For this review, take the finished solid that the model builds, in its own axes (mm). Round coordinates to 2 decimals unless told otherwise and drop trailing zeros. Write each loop counter-clockwise with the first axis right and the second up, starting at its lowest first coordinate (ties: lowest second). Pieces come first, ordered by that corner, then holes. Notation, with made-up numbers: M 61.25,70 L 103.25,70 A13 cw 103.25,88 Z; hole C 30,-11.75 d3. An arc over 180 degrees is marked long. One line per question, with ' | ' between items.
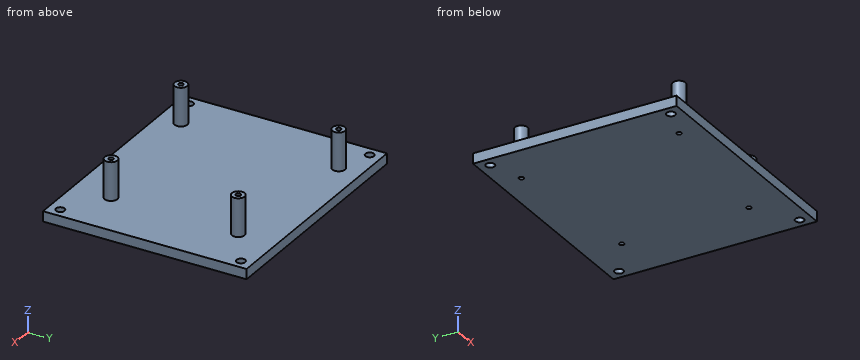
```python
from build123d import *

# Parameters (mm, degrees)
SKETCH_1_W          = 94
SKETCH_1_H          = 80
EXTRUDE_1_DEPTH     = 4
CUT_EXTRUDE_1_REACH = 63.847
SKETCH_2_R          = 1.7
SKETCH_3_R          = 2.5
EXTRUDE_2_DEPTH     = 15
CUT_EXTRUDE_2_REACH = 66.576
SKETCH_4_R          = 0.95


with BuildPart() as part:
    # 草图1 → 凸台-拉伸1 (new body)
    with BuildSketch(Plane.XY):
        Rectangle(SKETCH_1_W, SKETCH_1_H)
    extrude(amount=EXTRUDE_1_DEPTH)

    # 草图2 → 切除-拉伸1 (cut, up to next)
    with BuildSketch(Plane.XY.offset(4), mode=Mode.PRIVATE) as cut_extrude_1_sk1:
        with Locations((-43.1, -35.5)):
            Circle(SKETCH_2_R)
    cut_extrude_1_tool1 = extrude(cut_extrude_1_sk1.sketch, amount=-CUT_EXTRUDE_1_REACH, mode=Mode.PRIVATE) & part.part
    # 草图2 → 切除-拉伸1 (cut, up to next)
    with BuildSketch(Plane.XY.offset(4), mode=Mode.PRIVATE) as cut_extrude_1_sk2:
        with Locations((43.1, -35.5)):
            Circle(SKETCH_2_R)
    cut_extrude_1_tool2 = extrude(cut_extrude_1_sk2.sketch, amount=-CUT_EXTRUDE_1_REACH, mode=Mode.PRIVATE) & part.part
    # 草图2 → 切除-拉伸1 (cut, up to next)
    with BuildSketch(Plane.XY.offset(4), mode=Mode.PRIVATE) as cut_extrude_1_sk3:
        with Locations((43.1, 35.5)):
            Circle(SKETCH_2_R)
    cut_extrude_1_tool3 = extrude(cut_extrude_1_sk3.sketch, amount=-CUT_EXTRUDE_1_REACH, mode=Mode.PRIVATE) & part.part
    # 草图2 → 切除-拉伸1 (cut, up to next)
    with BuildSketch(Plane.XY.offset(4), mode=Mode.PRIVATE) as cut_extrude_1_sk4:
        with Locations((-43.1, 35.5)):
            Circle(SKETCH_2_R)
    cut_extrude_1_tool4 = extrude(cut_extrude_1_sk4.sketch, amount=-CUT_EXTRUDE_1_REACH, mode=Mode.PRIVATE) & part.part
    add(cut_extrude_1_tool1.solids().sort_by_distance((-43.1, -35.5, 4))[0], mode=Mode.SUBTRACT)
    add(cut_extrude_1_tool2.solids().sort_by_distance((43.1, -35.5, 4))[0], mode=Mode.SUBTRACT)
    add(cut_extrude_1_tool3.solids().sort_by_distance((43.1, 35.5, 4))[0], mode=Mode.SUBTRACT)
    add(cut_extrude_1_tool4.solids().sort_by_distance((-43.1, 35.5, 4))[0], mode=Mode.SUBTRACT)

    # 草图3 → 凸台-拉伸2 (add)
    with BuildSketch(Plane.XY.offset(4)):
        with Locations((-30, 31)):
            Circle(SKETCH_3_R)
        with Locations((-30, -31)):
            Circle(SKETCH_3_R)
        with Locations((27, 25)):
            Circle(SKETCH_3_R)
        with Locations((27, -25)):
            Circle(SKETCH_3_R)
    extrude(amount=EXTRUDE_2_DEPTH)

    # 草图4 → 切除-拉伸2 (cut, up to next)
    with BuildSketch(Plane.XY.offset(19), mode=Mode.PRIVATE) as cut_extrude_2_sk1:
        with Locations((-30, 31)):
            Circle(SKETCH_4_R)
    cut_extrude_2_tool1 = extrude(cut_extrude_2_sk1.sketch, amount=-CUT_EXTRUDE_2_REACH, mode=Mode.PRIVATE) & part.part
    # 草图4 → 切除-拉伸2 (cut, up to next)
    with BuildSketch(Plane.XY.offset(19), mode=Mode.PRIVATE) as cut_extrude_2_sk2:
        with Locations((27, 25)):
            Circle(SKETCH_4_R)
    cut_extrude_2_tool2 = extrude(cut_extrude_2_sk2.sketch, amount=-CUT_EXTRUDE_2_REACH, mode=Mode.PRIVATE) & part.part
    # 草图4 → 切除-拉伸2 (cut, up to next)
    with BuildSketch(Plane.XY.offset(19), mode=Mode.PRIVATE) as cut_extrude_2_sk3:
        with Locations((-30, -31)):
            Circle(SKETCH_4_R)
    cut_extrude_2_tool3 = extrude(cut_extrude_2_sk3.sketch, amount=-CUT_EXTRUDE_2_REACH, mode=Mode.PRIVATE) & part.part
    # 草图4 → 切除-拉伸2 (cut, up to next)
    with BuildSketch(Plane.XY.offset(19), mode=Mode.PRIVATE) as cut_extrude_2_sk4:
        with Locations((27, -25)):
            Circle(SKETCH_4_R)
    cut_extrude_2_tool4 = extrude(cut_extrude_2_sk4.sketch, amount=-CUT_EXTRUDE_2_REACH, mode=Mode.PRIVATE) & part.part
    add(cut_extrude_2_tool1.solids().sort_by_distance((-30, 31, 19))[0], mode=Mode.SUBTRACT)
    add(cut_extrude_2_tool2.solids().sort_by_distance((27, 25, 19))[0], mode=Mode.SUBTRACT)
    add(cut_extrude_2_tool3.solids().sort_by_distance((-30, -31, 19))[0], mode=Mode.SUBTRACT)
    add(cut_extrude_2_tool4.solids().sort_by_distance((27, -25, 19))[0], mode=Mode.SUBTRACT)


solid = part.part
```
Item 1: Take a section at D-D (x = 10.5). Write out the cut boundary in (y, z), then the cut area to 3 significant figures.
Results:
outline: M -40,0 L 40,0 L 40,4 L -40,4 Z | area: 320 mm2
Item 2: To check wall thickness, follow line 1 along Y through (x, z) = (27, 4.5); line 2 along Y through (x, z) = (-30, 9); line 3 along Y through (x, z) = (43.1, 3.1). State the ranges of each line that lie inside material, in increasing order. Write a range as from..to.
Results:
line 1: -27.5..-25.95, -24.05..-22.5, 22.5..24.05, 25.95..27.5 | line 2: -33.5..-31.95, -30.05..-28.5, 28.5..30.05, 31.95..33.5 | line 3: -40..-37.2, -33.8..33.8, 37.2..40
Item 3: Take a section at C-C (y = 3). Write out the cut boundary in (x, z), then the cut area to 3 significant figures.
Results:
outline: M -47,0 L 47,0 L 47,4 L -47,4 Z | area: 376 mm2
Item 4: Take a section at A-A (y = -35.5). Write out the cut boundary in (x, z).
Results:
outline: M -47,0 L -44.8,0 L -44.8,4 L -47,4 Z; M -41.4,0 L 41.4,0 L 41.4,4 L -41.4,4 Z; M 44.8,0 L 47,0 L 47,4 L 44.8,4 Z
Item 5: Insertion check: pin 1 Ø24 at (x, y) = (15.5, 3.5) entering from +Z; pin 2 Ø6 at (x, z) = (-34.5, 14) entering from +Y; pin 3 Ø5 at (y, z) = (-28.5, 14.5) entering from -X; pin 4 Ø2.5 at (x, y) = (43.1, -35.5) entering from -Z. Each pin has a flat end and moves straight along its axis. Give the tip position at first contact, or say it passes through.
Results:
pin 1: z = 4 | pin 2: y = 33 | pin 3: x = -32.5 | pin 4: through
Item 6: Take a section at B-B (x = 43.1). Write out the cut boundary in (y, z), then the cut area to 3 significant figures.
Results:
outline: M -40,0 L -37.2,0 L -37.2,4 L -40,4 Z; M -33.8,0 L 33.8,0 L 33.8,4 L -33.8,4 Z; M 37.2,0 L 40,0 L 40,4 L 37.2,4 Z | area: 293 mm2
